CAD build for the part. Positions are in the model's coordinates, mm. A direction names the side the tool comes from. Round coordinates to 2 decimals unless told otherwise and drop trailing zeros. Write each loop counter-clockwise with the first axis right and the second up, starting at its lowest first coordinate (ties: lowest second). Pieces come first, ordered by that corner, then holes. Notation, with made-up numbers: (78, 5) - (87, 5) arc R19 ccw to (87, 31) - close; hole circle Ø6 at (24.25, -12). An arc over 180 degrees is marked (long way). Put each result on its own line as item: value. Start each with the question number.
Item 1: Cut at B-B (y = 28.5). Give the cut face in (x, z).
Item 2: Drill centre lines: line 1 (X direction, y = 3.25, z = 0); line 2 (X direction, y = 8, z = 0) (3 decimals); line 3 (X direction, y = 54, z = 0) (3 decimals). Where is each one in solid material? Low to high. Write a range as from..to.
Item 3: Mould opens along Z. For faces 1 (the flat face through (16, 59, 0)), 2 (the cylindrical face through (5.592, 3.341, 13.487)) say: released by +Z, released by -Z, zero draft, split by the parting line, or undercut.
Item 4: Pin check, flat tips, straight feed: pin 1 Ø1 at (x, y) = (12.5, 11.5) entering from +Z; pin 2 Ø4 at (x, z) = (-19.5, 0) entering from -Y; pin 3 Ø16 at (x, z) = (0, 0) entering from -Y; pin 4 Ø1 at (x, y) = (1.5, 16) entering from +Z. Stop position of each tip, or through.
Item 5: 3-axis set-ups, long thin cutter, end or side, ignore diameter. For faces 3 (the cylindrical face through (-13.906, 54.299, -1.826)), 4 (the flat face through (12, 2.7, 8)): which of +Z, -Z, +X, -X, +Y, -Y reach the whole face in a straight line?
Item 6: Cut at A-A (y = 52.5). Give the cut face in (x, z) (3 decimals), and give its area (3 significant figures).
```python
from build123d import *

# Parameters (mm, degrees)
ZKOSEN_1_SIZE   = 1
M6_Z_VIT1_D     = 5
M6_Z_VIT1_DEPTH = 12
M6_Z_VIT1_TIP   = 1.502151548
ZKOSEN_2_SIZE   = 1
ZKOSEN_3_SIZE   = 0.5


with BuildPart() as part:
    # Skica1 → Rotovat1 (revolve)
    with BuildSketch(Plane.XY, mode=Mode.PRIVATE) as rotovat1_sk:
        Polygon((-25, 0), (-25, 59), (-14.025, 59), (-14.025, 50.7), (-10, 50.7), (-10, 11.999895833), (-14.025, 11.999895833), (-14.025, 3.999895833), (-14.6, 3.999895833), (-14.6, 2.699895833), (-13.975, 2.699895833), (-13.975, 0), align=None)
    revolve(rotovat1_sk.sketch.rotate(Axis((0, 0, 0), (0, -1, 0)), 270), axis=Axis((0, 0, 0), (0, -1, 0)))

    # Zkosení1
    zkosen_1_edges = [part.edges().sort_by_distance(p)[0] for p in [
        (0, 11.999895833, -10),
        (0, 50.7, -10),
        (0, 59, -14.025),
        (0, 0, -13.975),
    ]]
    chamfer(zkosen_1_edges, length=ZKOSEN_1_SIZE)

    # M6 závit1
    with Locations(Plane(origin=(0, 0, 0), x_dir=(-1, 0, 0), z_dir=(0, -1, 0))):
        with Locations((0, 19.5), (19.5, 0), (0, -19.5), (-19.5, 0)):
            Hole(M6_Z_VIT1_D / 2, depth=M6_Z_VIT1_DEPTH)
            with Locations((0, 0, -(M6_Z_VIT1_DEPTH + M6_Z_VIT1_TIP / 2))):  # 118° drill point
                Cone(0, M6_Z_VIT1_D / 2, M6_Z_VIT1_TIP, mode=Mode.SUBTRACT)

    # Zkosení2
    zkosen_2_edges = [part.edges().sort_by_distance(p)[0] for p in [
        (0, 59, -25),
        (0, 0, -25),
    ]]
    chamfer(zkosen_2_edges, length=ZKOSEN_2_SIZE)

    # Zkosení3
    zkosen_3_edges = [part.edges().sort_by_distance(p)[0] for p in [
        (17, 0, 0),
        (-2.5, 0, 19.5),
        (-22, 0, 0),
        (-2.5, 0, -19.5),
    ]]
    chamfer(zkosen_3_edges, length=ZKOSEN_3_SIZE)


solid = part.part
```
Output values:
1. outline: circle Ø50 at (0, 0); hole circle Ø20 at (0, 0)
2. line 1: -25..-22, -17..-14.6, 14.6..17, 22..25
2. line 2: -25..-22, -17..-14.025, 14.025..17, 22..25
2. line 3: -25..-14.025, 14.025..25
3. face 1: zero draft
3. face 2: undercut
4. pin 1: z = 21.93
4. pin 2: y = 12.3
4. pin 3: through
4. pin 4: z = 24.98
5. face 3: +Y
5. face 4: none
6. outline: circle Ø50 at (0, 0); hole circle Ø28.05 at (0, 0)
6. area: 1,350 mm2
